The model under review builds one solid part; all positions refer to its coordinate system, in mm. Round coordinates to 2 decimals unless told otherwise and drop trailing zeros. Loops run counter-clockwise (first coordinate to the right, second up) from the corner with the lowest first, then second, coordinate; pieces in that order, holes last. Notation, with made-up numbers: M 40.25,64.25 L 99.25,64.25 A26 cw 99.25,100.25 Z; hole C 73,82 d11. An arc over 180 degrees is marked long. Answer in a Markdown table with one row per item. Add a question column.
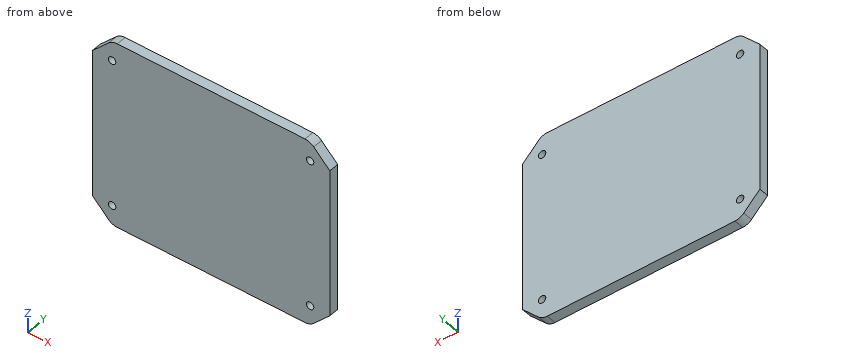
from build123d import *

# Parameters (mm, degrees)
SKETCH1_R           = 1.5
BOSS_EXTRUDE1_DEPTH = 4


with BuildPart() as part:
    # Sketch1 → Boss-Extrude1 (new body)
    with BuildSketch(Plane(origin=(0, 0, 0), x_dir=(1, 0, 0), z_dir=(0, 1, 0))):
        with BuildLine():
            Line((-40.245236531, 36.750583468), (-46.780770437, 30.215049562))
            Line((-46.780770437, 30.215049562), (-46.780770437, -29.784950438))
            Line((-46.780770437, -29.784950438), (-40.245236531, -36.320484344))
            ThreePointArc((-40.245236531, -36.320484344), (-38.623119787, -37.4043481), (-36.709702625, -37.784950438))
            Line((-36.709702625, -37.784950438), (39.290297375, -37.784950438))
            ThreePointArc((39.290297375, -37.784950438), (41.203714536, -37.4043481), (42.82583128, -36.320484344))
            Line((42.82583128, -36.320484344), (49.361365186, -29.784950438))
            Line((49.361365186, -29.784950438), (49.361365186, 30.215049562))
            Line((49.361365186, 30.215049562), (42.82583128, 36.750583468))
            ThreePointArc((42.82583128, 36.750583468), (41.203714536, 37.834447225), (39.290297375, 38.215049562))
            Line((39.290297375, 38.215049562), (-36.709702625, 38.215049562))
            ThreePointArc((-36.709702625, 38.215049562), (-38.623119787, 37.834447225), (-40.245236531, 36.750583468))
        make_face()
        with Locations(Location((41.361365186, -29.784950438, 0), (0, 0, 270))):
            Circle(SKETCH1_R, mode=Mode.SUBTRACT)
        with Locations(Location((41.361365186, 30.215049562, 0), (0, 0, 270))):
            Circle(SKETCH1_R, mode=Mode.SUBTRACT)
        with Locations(Location((-38.780770437, -29.784950438, 0), (0, 0, 270))):
            Circle(SKETCH1_R, mode=Mode.SUBTRACT)
        with Locations(Location((-38.780770437, 30.215049562, 0), (0, 0, 270))):
            Circle(SKETCH1_R, mode=Mode.SUBTRACT)
    extrude(amount=BOSS_EXTRUDE1_DEPTH)


solid = part.part
1. Take a section at B-B, the plane z = 33. State the section outline as (x, y) points.
2. Take a section at A-A, the plane y = 0.9. State the section outline as (x, z) points, and give its area (3 significant figures).
3. To check wall thickness, follow probe 1 along X at (y, z) = (3.6, 28.5); probe 2 along Z at (x, y) = (44, 2.7). State the ranges of each line that lie inside material, in increasing order.
4. For pin 1 Ø3.5 at (x, z) = (41.36, 29.78) entering from +Y, flat-tipped, find the tip position at first contact; note if it passes through.
Check sheet entries:
| question | item | result |
|---|---|---|
| 1 | outline | M -43.57,0 L 46.15,0 L 46.15,4 L -43.57,4 Z |
| 2 | outline | M -46.78,-30.22 L -40.25,-36.75 A5 ccw -36.71,-38.22 L 39.29,-38.22 A5 ccw 42.83,-36.75 L 49.36,-30.22 L 49.36,29.78 L 42.83,36.32 A5 ccw 39.29,37.78 L -36.71,37.78 A5 ccw -40.25,36.32 L -46.78,29.78 Z; hole C -38.78,-30.22 d3; hole C -38.78,29.78 d3; hole C 41.36,-30.22 d3; hole C 41.36,29.78 d3 |
| 2 | area | 7,150 mm^2 |
| 3 | probe 1 | x = -46.78 to -39.55, -38.01 to 40.59, 42.14 to 49.36 |
| 3 | probe 2 | z = -35.58 to 35.15 |
| 4 | pin 1 | stops at y = 4 |
